Autodesk Inventor part; units mm, degrees
ref_plane "YZ Plane" through (0, 0, 0) normal (1, 0, 0) x (0, 1, 0)
ref_plane "XZ Plane" through (0, 0, 0) normal (0, 1, 0) x (-1, 0, 0)
ref_plane "XY Plane" through (0, 0, 0) normal (0, 0, 1) x (1, 0, 0)
sketch "Skizze1" plane through (0, 0, 0) normal (0, 0, 1) x (1, 0, 0)
  line L0 (15.5, 18) -> (16.5, 18)
  line L1 (16.5, 18) -> (16.5, 5)
  line L2 (11.5, 0) -> (0, 0)
  line L3 (0, 0) -> (0, 1)
  line L4 (0, 1) -> (11, 1)
  line L5 (15.5, 5.5) -> (15.5, 15)
  line L6 (15.5, 15) -> (13.5, 15)
  line L7 (13.5, 15) -> (13.5, 15.5)
  line L8 (13.5, 15.5) -> (15.5, 18)
  arc A0 (11, 1) -> (15.5, 5.5) centre (11, 5.5) ccw
  arc A1 (11.5, 0) -> (16.5, 5) centre (11.5, 5) ccw
  point P0 (16.5, 0)
  point P1 (15.5, 1)
  point P2 (16, 18)
  dimension "d0" = 1
  dimension "d1" = 1
  dimension "d2" = 15.5
  dimension "d3" = 14
  dimension "d4" = 3
  dimension "d5" = 0.5
  dimension "d6" = 1
  dimension "d7" = 2
  dimension "d10" = 4.5
  dimension "d11" = 5
extrude "Extrusion1" add sketch "Skizze1" along normal blind 15
mirror "Spiegeln1" about plane through (0, 0, 0) normal (1, 0, 0)
properties part number "P_Halter"
Verification items for the finished model (mm, model axes). A direction names the side the tool comes from. Coordinates: 2 decimals unless noted, no trailing zeros. Write each loop counter-clockwise with the first axis right and the second up, starting at its lowest first coordinate (ties: lowest second). Pieces come first, ordered by that corner, then holes. Notation, with made-up numbers: M 26.5,3.25 L 77.5,3.25 A20 ccw 77.5,28.25 Z; hole C 26,-7.5 d3. An arc over 180 degrees is marked long. Answer as a JSON object with one key per item and string values. Group by question number.
(1) Cross-section at C-C, the plane x = 14. Record the cut outline in (y, z) (3 decimals), and give its area (3 significant figures).
(2) Gauge pin test, flat ends, axial feed: pin 1 (5 mm diameter, centred on x = -3.5, z = 6.5, fed in from +Y); pin 2 (1.6 mm diameter, centred on x = 14, z = 8.5, fed in from -Y); pin 3 (10 mm diameter, centred on x = -2, y = 10, fed in from +Z); pin 4 (1 mm diameter, centred on x = -14, z = 6, fed in from -Y). Record the tip position at first contact, or that the pin passes through.
(3) Release check for a two-part mould opening along X. For faces 1 (the face through (16.5, 12, 7)), 2 (the face through (-15.5, 10, 7)), 3 (the face through (14.486, 16.732, 7.395)), 4 (the face through (16, 18, 7)) record: +X half, -X half, draft (parallel to the pull), parting line (faces both ways), or undercut.
(4) Material ranges on line 1 (X direction, y = 10.5, z = 6.75); line 2 (X direction, y = 15.5, z = 9.25); line 3 (Y direction, x = -6, z = 5.5), recorded low to high.
(5) Cross-section at B-B, the plane z = 3. Record the cut outline in (x, y), and give its area (3 significant figures).
(6) Tool access check on faces 5 (the face through (-14.147, 2.283, 7.395)), 6 (the face through (0, 1, 7)), 7 (the face through (-16, 18, 7)). Record the directions out of +Z, -Z, +X, -X, +Y, -Y that give a thin tool (end or side, any length) a straight path to the whole face; none if there is none.
(7) Cross-section at A-A, the plane y = 11.25. Record the cut outline in (x, z), and give its area (3 significant figures).
(8) Cross-section at D-D, the plane x = 6. Record the cut outline in (y, z), and give its area (3 significant figures).
Reply:
{
 "1": {"outline": "M 0.67,0 L 2.146,0 L 2.146,15 L 0.67,15 Z; M 15,0 L 16.125,0 L 16.125,15 L 15,15 Z", "area": "39.0 mm²"},
 "2": {"pin 1": "y = 1", "pin 2": "y = 0.3", "pin 3": "through", "pin 4": "y = 0.42"},
 "3": {"face 1": "+X half", "face 2": "undercut", "face 3": "undercut", "face 4": "draft"},
 "4": {"line 1": "-16.5 to -15.5, 15.5 to 16.5", "line 2": "-16.5 to -13.5, 13.5 to 16.5", "line 3": "0 to 1"},
 "5": {"outline": "M -16.5,5 A5 ccw -11.5,0 L 11.5,0 A5 ccw 16.5,5 L 16.5,18 L 15.5,18 L 13.5,15.5 L 13.5,15 L 15.5,15 L 15.5,5.5 A4.5 cw 11,1 L -11,1 A4.5 cw -15.5,5.5 L -15.5,15 L -13.5,15 L -13.5,15.5 L -15.5,18 L -16.5,18 Z", "area": "72.0 mm²"},
 "6": {"face 5": "+Z, -Z", "face 6": "+Z, -Z, +Y", "face 7": "+Z, -Z, +X, -X, +Y"},
 "7": {"outline": "M -16.5,0 L -15.5,0 L -15.5,15 L -16.5,15 Z; M 15.5,0 L 16.5,0 L 16.5,15 L 15.5,15 Z", "area": "30.0 mm²"},
 "8": {"outline": "M 0,0 L 1,0 L 1,15 L 0,15 Z", "area": "15.0 mm²"}
}
